Here's how the part is built. I have some questions about the finished solid (model axes, mm). Face numbers are marked on the shaded views. A direction names the side the tool comes from. Round coordinates to 2 decimals unless told otherwise and drop trailing zeros. Order: outer loops, then holes, each group sorted by start corner. A loop starts at its lowest first (then second) coordinate and runs counter-clockwise, first axis right, second up. Notation, with made-up numbers: (-22, 14.5) - (18, 14.5) arc R17 ccw to (18, 27.5) - close; hole circle Ø1 at (-10.5, -17). An arc over 180 degrees is marked (long way). Answer as a JSON object with one key per item and string values.
```python
from build123d import *

# Parameters (mm, degrees)
SKETCH1_W           = 12.7
SKETCH1_H           = 44.45
BOSS_EXTRUDE1_DEPTH = 127
SKETCH2_R           = 6.35
CUT_EXTRUDE1_DEPTH  = 142.028625197
SKETCH4_W           = 88.9
SKETCH4_H           = 57.15
CUT_EXTRUDE2_DEPTH  = 147.187978302


with BuildPart() as part:
    # Sketch1 → Boss-Extrude1 (new body)
    with BuildSketch(Plane.YZ):
        with BuildLine():
            ThreePointArc((15.875, -38.1), (8.435512242, -20.139487758), (-9.525, -12.7))
            Line((-9.525, -12.7), (-9.525, 0))
            Line((-9.525, 0), (0, 0))
            Line((0, 0), (0, 44.45))
            Line((0, 44.45), (12.7, 44.45))
            Line((12.7, 44.45), (12.7, 0))
            Line((12.7, 0), (34.925, -19.098767483))
            Line((34.925, -19.098767483), (34.925, -57.15))
            Line((34.925, -57.15), (15.875, -57.15))
            Line((15.875, -57.15), (15.875, -38.1))
        make_face()
        with Locations((6.35, 22.225)):
            Rectangle(SKETCH1_W, SKETCH1_H)
    extrude(amount=-BOSS_EXTRUDE1_DEPTH)

    # Sketch2 → Cut-Extrude1 (cut, through all)
    with BuildSketch(Plane(origin=(0, 12.7, 0), x_dir=(-1, 0, 0), z_dir=(0, 1, 0))):
        with BuildLine():
            Line((101.6, 31.75), (127, 31.75))
            Line((127, 31.75), (127, 44.45))
            Line((127, 44.45), (12.700000053, 44.45))
            ThreePointArc((12.700000053, 44.45), (21.68025614, 40.730256102), (25.4, 31.75))
            Line((25.4, 31.75), (25.4, 19.05))
            Line((25.4, 19.05), (101.6, 19.05))
            Line((101.6, 19.05), (101.6, 31.75))
        make_face()
        with BuildLine():
            ThreePointArc((0, 31.75), (3.719743898, 40.73025614), (12.700000053, 44.45))
            Line((12.700000053, 44.45), (0, 44.45))
            Line((0, 44.45), (0, 31.75))
        make_face()
        with Locations(Location((12.7, 31.75, 0), (0, 0, 90))):
            Circle(SKETCH2_R)
    extrude(amount=-CUT_EXTRUDE1_DEPTH, mode=Mode.SUBTRACT)

    # Sketch4 → Cut-Extrude2 (cut, through all)
    with BuildSketch(Plane(origin=(0, 34.925, 0), x_dir=(-1, 0, 0), z_dir=(0, 1, 0))):
        with Locations((63.5, -28.575)):
            Rectangle(SKETCH4_W, SKETCH4_H)
    extrude(amount=-CUT_EXTRUDE2_DEPTH, mode=Mode.SUBTRACT)

    # Mirror1: part across plane


with BuildPart() as part_1:
    add(part.part)
    add(part.part.mirror(Plane(origin=(-127, -9.525, 0), x_dir=(0, 0, 1), z_dir=(0, -1, 0))))


solid = part_1.part
```
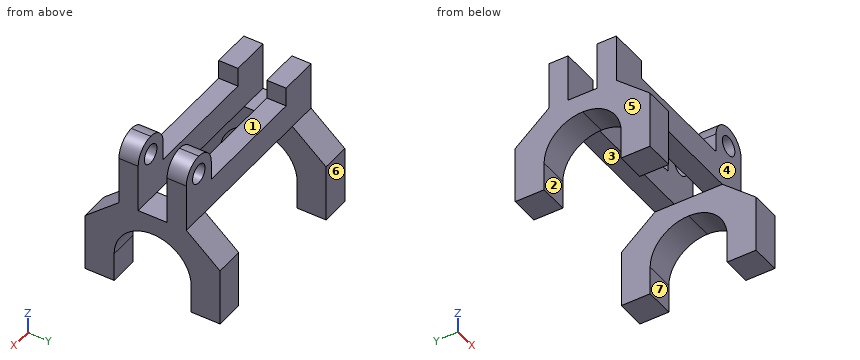
1. Imagine slicing it at C-C (y = -25). List the corners of the cut face in (x, z) for me, plus the area to 3 significant figures.
Responses:
{"outline": "(-127, -17.96) - (-107.95, -17.96) - (-107.95, 0) - (-19.05, 0) - (-19.05, -17.96) - (0, -17.96) - (0, 31.75) arc R12.7 ccw to (-25.4, 31.75) - (-25.4, 19.05) - (-101.6, 19.05) - (-101.6, 31.75) - (-127, 31.75) - close; hole circle Ø12.7 at (-12.7, 31.75)", "area": "3,880 mm2"}
2. Imagine slicing it at D-D (z = -33.5). List the corners of the cut face in (x, y) for me (3 decimals), plus the area to 3 significant figures.
Responses:
{"outline": "(-127, -53.975) - (-107.95, -53.975) - (-107.95, -34.505) - (-127, -34.505) - close; (-127, 15.455) - (-107.95, 15.455) - (-107.95, 34.925) - (-127, 34.925) - close; (-19.05, -53.975) - (0, -53.975) - (0, -34.505) - (-19.05, -34.505) - close; (-19.05, 15.455) - (0, 15.455) - (0, 34.925) - (-19.05, 34.925) - close", "area": "1,480 mm2"}
3. Thinking about a two-plate mould opening in Y: for the marked faces 4, 5, 6 and 7, which applies, pulls with the +Y half, pulls with the -Y half, needs draft (parallel to the pull), parting line crosses it, or undercut?
Responses:
{"face 4": "pulls with the -Y half", "face 5": "needs draft", "face 6": "pulls with the +Y half", "face 7": "undercut"}
4. For P1, Ø22, axis at x = -79, z = 19, coming from the +Y side; P2, Ø21, axis at x = -117, y = -8, coming from the +Z side; P3, Ø12, axis at x = -21.5, y = -43.5, coming from the +Z side; P4, Ø6, axis at y = -16, z = -17, coming from the +X side, each with a flat end and sliding along its axis, tell me the tip position at first contact or that it passes through.
Responses:
{"P1": "y = 12.7", "P2": "z = 31.75", "P3": "z = -5.39", "P4": "through"}
5. If I drill on L1, parallel to Y at x = -92, z = 17; L2, parallel to X at y = -38, z = -53; L3, parallel to Y at x = -118, z = -47.5 (3 decimals), over which ranges is the centre line in solid material (lowest first)? Write a range as [from, to].
Responses:
{"L1": "[-31.75, -19.05], [0, 12.7]", "L2": "[-127, -107.95], [-19.05, 0]", "L3": "[-53.975, -34.925], [15.875, 34.925]"}
6. Imagine slicing it at B-B (y = 23.5). List the corners of the cut face in (x, z) for me.
Responses:
{"outline": "(-127, -57.15) - (-107.95, -57.15) - (-107.95, -9.28) - (-127, -9.28) - close; (-19.05, -57.15) - (0, -57.15) - (0, -9.28) - (-19.05, -9.28) - close"}
7. For the marked faces 1, 2 and 3, which set-ups out of +Z, -Z, +X, -X, +Y, -Y let a thin tool reach every point of the face, with its end or its side?
Responses:
{"face 1": "+Z, +Y, -Y", "face 2": "-Z, +X, -X", "face 3": "-Z, +Y, -Y"}
8. Imagine slicing it at A-A (x = -92). List the corners of the cut face in (y, z) for me, plus the area to 3 significant figures.
Responses:
{"outline": "(-31.75, 0) - (-19.05, 0) - (-19.05, 19.05) - (-31.75, 19.05) - close; (0, 0) - (12.7, 0) - (12.7, 19.05) - (0, 19.05) - close", "area": "484 mm2"}
